```python
from build123d import *

# Parameters (mm, degrees)
F1_DEPTH = 25.4
F2_R     = 6.35
F3_DEPTH = 25.4
F5_DEPTH = 25.4
F7_DEPTH = 12.701


with BuildPart() as f1:
    # F0 (on Front) → F1 (new body)
    with BuildSketch(Plane.XZ):
        with BuildLine():
            Line((-47.538182, 38.1), (-47.538182, 0))
            Line((-47.538182, 0), (22.311818, 0))
            Line((22.311818, 0), (22.311818, 12.7))
            Line((22.311818, 12.7), (-22.138182, 12.7))
            Line((-22.138182, 12.7), (-22.138182, 38.1))
            ThreePointArc((-22.138182, 38.1), (-34.838182, 50.8), (-47.538182, 38.1))
        make_face()
    extrude(amount=F1_DEPTH)

    # F2 (on face) → F3 (cut)
    with BuildSketch(Plane.XZ.offset(25.4)):
        with Locations((-34.838182, 38.1)):
            Circle(F2_R)
    extrude(amount=-F3_DEPTH, mode=Mode.SUBTRACT)

    # F4 (on face) → F5 (cut)
    with BuildSketch(Plane.XY.offset(12.7)):
        with BuildLine():
            ThreePointArc((9.611818, 0), (18.592074, -3.719744), (22.311818, -12.7))
            Line((22.311818, -12.7), (22.311818, 0))
            Line((22.311818, 0), (9.611818, 0))
        make_face()
        with BuildLine():
            ThreePointArc((22.311818, -12.7), (18.592074, -21.680256), (9.611818, -25.4))
            Line((9.611818, -25.4), (22.311818, -25.4))
            Line((22.311818, -25.4), (22.311818, -12.7))
        make_face()
    extrude(amount=-F5_DEPTH, mode=Mode.SUBTRACT)

    # F6 (on face) → F7 (cut, through all)
    with BuildSketch(Plane.XY.offset(12.7)):
        with BuildLine():
            ThreePointArc((-12.100862, -18.09319), (-7.610734, -16.233318), (-5.750862, -11.74319))
            ThreePointArc((-5.750862, -11.74319), (-7.610734, -7.253062), (-12.100862, -5.39319))
            Line((-12.100862, -5.39319), (-12.100862, -18.09319))
        make_face()
        with BuildLine():
            Line((-12.100862, -18.09319), (-12.100862, -5.39319))
            ThreePointArc((-12.100862, -5.39319), (-18.450862, -11.74319), (-12.100862, -18.09319))
        make_face()
        with BuildLine():
            ThreePointArc((-12.100862, -5.39319), (-7.610734, -7.253062), (-5.750862, -11.74319))
            ThreePointArc((-5.750862, -11.74319), (-7.610734, -16.233318), (-12.100862, -18.09319))
            Line((-12.100862, -18.09319), (6.949138, -18.09319))
            ThreePointArc((6.949138, -18.09319), (0.599138, -11.74319), (6.949138, -5.39319))
            Line((6.949138, -5.39319), (-12.100862, -5.39319))
        make_face()
        with BuildLine():
            Line((6.949138, -18.09319), (6.949138, -5.39319))
            ThreePointArc((6.949138, -5.39319), (0.599138, -11.74319), (6.949138, -18.09319))
        make_face()
        with BuildLine():
            ThreePointArc((13.299138, -11.74319), (11.439266, -7.253062), (6.949138, -5.39319))
            Line((6.949138, -5.39319), (6.949138, -18.09319))
            ThreePointArc((6.949138, -18.09319), (11.439266, -16.233318), (13.299138, -11.74319))
        make_face()
    extrude(amount=-F7_DEPTH, mode=Mode.SUBTRACT)


solid = f1.part
```
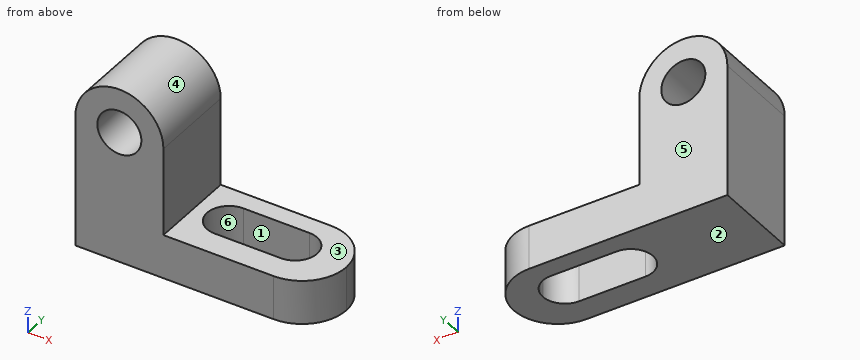
Check sheet for the modelled part. Datum: model origin and axes. Units: mm. Face numbers are marked on the shaded views. A direction names the side the tool comes from. Coordinates: 2 decimals unless noted, no trailing zeros. Write each loop counter-clockwise with the first axis right and the second up, starting at its lowest first coordinate (ties: lowest second). Pieces come first, ordered by that corner, then holes. Notation, with made-up numbers: M 22,21 L 52,21 A26 cw 52,40 Z; hole C 73.25,47.25 d2. An arc over 180 degrees is marked long. Use one line per item in the form item = value.
Item 1: Sectioned sample at A-A, the plane x = 2. Record the cut outline in (y, z), and give its area (3 significant figures).
Answer below:
outline = M -25.4,0 L -18.09,0 L -18.09,12.7 L -25.4,12.7 Z; M -5.39,0 L 0,0 L 0,12.7 L -5.39,12.7 Z
area = 161 mm^2
Item 2: Sectioned sample at D-D, the plane y = -21. Record the cut outline in (x, z), and give its area (3 significant figures).
Answer below:
outline = M -47.54,0 L 19.22,0 L 19.22,12.7 L -22.14,12.7 L -22.14,38.1 A12.7 ccw -47.54,38.1 Z; hole C -34.84,38.1 d12.7
area = 1,620 mm^2
Item 3: Set-up check for the marked faces 1, 2 and 3: record each of +Z, -Z, +X, -X, +Y, -Y from which the full face is reachable in a straight line by a thin tool's end or side.
Answer below:
face_1 = +Z, -Z
face_2 = -Z, +X, -X, +Y, -Y
face_3 = +Z, +X, +Y, -Y
Item 4: Sectioned sample at C-C, the plane z = 6. Record the cut outline in (x, y).
Answer below:
outline = M -47.54,-25.4 L 9.61,-25.4 A12.7 ccw 9.61,0 L -47.54,0 Z; hole M -12.1,-18.09 L 6.95,-18.09 A6.35 ccw 6.95,-5.39 L -12.1,-5.39 A6.35 ccw Z
Item 5: Gauge pin test, flat ends, axial feed: pin 1 Ø1 at (y, z) = (-5.5, 38) entering from +X; pin 2 Ø1 at (x, z) = (-2.5, 15) entering from -Y; pin 3 Ø12 at (y, z) = (-11.5, 11.5) entering from +X; pin 4 Ø1 at (x, y) = (-10, -20) entering from +Z. Record the tip position at first contact, or that the pin passes through.
Answer below:
pin_1 = -22.14
pin_2 = through
pin_3 = 22.31
pin_4 = 12.7
Item 6: Material ranges on L1, parallel to Y at x = -11, z = 5.5; L2, parallel to X at y = -6, z = 41.5; L3, parallel to Z at x = -14, y = -18, recorded low to high. Write a range as from..to.
Answer below:
L1 = -25.4..-18.09, -5.39..0
L2 = -47.07..-40.2, -29.48..-22.6
L3 = 0..12.7
Item 7: Release check for a two-part mould opening along X. For the marked faces 4, 5 and 6 record: pulls with the +X half, pulls with the -X half, needs draft (parallel to the pull), parting line crosses it, or undercut.
Answer below:
face_4 = parting line crosses it
face_5 = needs draft
face_6 = undercut
Item 8: Sectioned sample at B-B, the plane y = -14.5. Record the cut outline in (x, z), and give its area (3 significant figures).
Answer below:
outline = M -47.54,0 L -17.82,0 L -17.82,12.7 L -22.14,12.7 L -22.14,38.1 A12.7 ccw -47.54,38.1 Z; M 12.67,0 L 22.18,0 L 22.18,12.7 L 12.67,12.7 Z; hole C -34.84,38.1 d12.7
area = 1,270 mm^2
